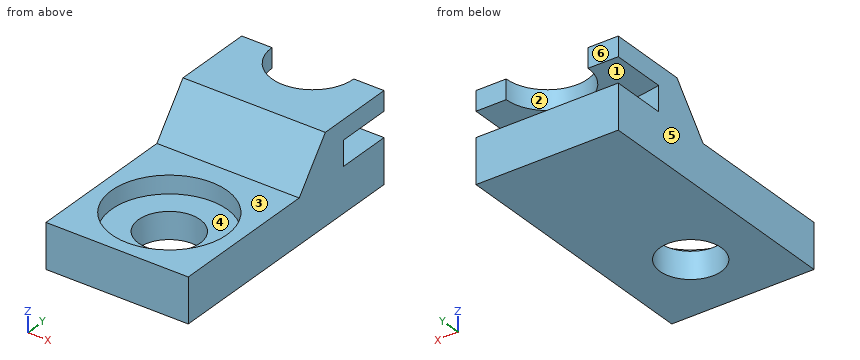
```python
from build123d import *

# Parameters (mm, degrees)
F0_W           = 10.16
F0_H           = 19.05
F1_DEPTH       = 3.175
F4_DEPTH       = 10.16
F6_D           = 4.4
F6_DEPTH       = 12.7
F6_CBORE_D     = 8.25
F6_CBORE_DEPTH = 1.27
F7_R           = 25.4
F8_DEPTH       = 1.778
F9_R           = 2.921
F10_DEPTH      = 2.54


with BuildPart() as f1:
    # F0 (on Top) → F1 (new body)
    with BuildSketch(Plane.XY):
        Rectangle(F0_W, F0_H)
    extrude(amount=F1_DEPTH)

    # F2 (on face) → F4 (join, through all)
    with BuildSketch(Plane.YZ.offset(5.08)):
        Polygon((3.81, 6.35), (1.27, 3.175), (9.525, 3.175), (9.525, 6.35), align=None)
    extrude(amount=-F4_DEPTH)

    # F6
    with Locations(Plane.XY.offset(3.175)):
        with Locations((0, -4.445)):
            CounterBoreHole(F6_D / 2, F6_CBORE_D / 2, F6_CBORE_DEPTH, depth=F6_DEPTH)

    # F7 (on face) → F8 (cut)
    with BuildSketch(Plane.XY.offset(3.175)):
        with Locations((0, 30.48)):
            Circle(F7_R)
    extrude(amount=F8_DEPTH, mode=Mode.SUBTRACT)

    # F9 (on face) → F10 (cut)
    with BuildSketch(Plane.XY.offset(6.35)):
        with Locations((0, 9.525)):
            Circle(F9_R)
    extrude(amount=-F10_DEPTH, mode=Mode.SUBTRACT)


solid = f1.part
```
Input: part model. Units: mm. Frame: model coordinates. Face numbers are marked on the shaded views. A direction names the side the tool comes from. Round coordinates to 2 decimals unless told otherwise and drop trailing zeros. Loops run counter-clockwise (first coordinate to the right, second up) from the corner with the lowest first, then second, coordinate; pieces in that order, holes last. Notation, with made-up numbers: (72.5, 60) -> (98.5, 60) arc R8 ccw to (98.5, 73) -> close; hole circle Ø8 at (84, -26.5). An arc over 180 degrees is marked (long way). Write each question's results on one line, items separated by ' | '.
1. Mould query, pull axis Y, two halves, no side actions, for the marked faces 4, 5 and 6. Classes: +Y half, -Y half, draft (parallel to the pull), parting line (faces both ways), or undercut.
Geometry results:
face 4: undercut | face 5: draft | face 6: +Y half
2. First-contact query: P1, Ø4, axis at x = 0, y = -4.5, coming from the +Z side; P2, Ø5, axis at x = 1.5, y = -6.5, coming from the +Z side (3 decimals). Flat tips, straight axial feed; report the tip coordinate or a pass-through.
Geometry results:
P1: through | P2: z = 3.175
3. Section C-C (x = -3.5). Return loops of the section in (y, z) (3 decimals), and give its area (3 significant figures).
Geometry results:
outline: (-9.525, 0) -> (9.525, 0) -> (9.525, 3.175) -> (5.322, 3.175) -> (5.322, 4.953) -> (9.525, 4.953) -> (9.525, 6.35) -> (3.81, 6.35) -> (1.27, 3.175) -> (-2.262, 3.175) -> (-2.262, 1.905) -> (-6.628, 1.905) -> (-6.628, 3.175) -> (-9.525, 3.175) -> close | area: 69.6 mm2
4. Section B-B (y = 7.5). Return loops of the section in (x, z) (3 decimals).
Geometry results:
outline: (-5.08, 0) -> (5.08, 0) -> (5.08, 3.175) -> (-5.08, 3.175) -> close; (-5.08, 4.953) -> (-2.105, 4.953) -> (-2.105, 6.35) -> (-5.08, 6.35) -> close; (2.105, 4.953) -> (5.08, 4.953) -> (5.08, 6.35) -> (2.105, 6.35) -> close
5. Ray query, line 1 (Z direction, x = 4.5, y = -4.75) (3 decimals); line 2 (Y direction, x = 0, z = 0.5) (3 decimals); line 3 (Y direction, x = -3.25, z = 2.75) (3 decimals). Return the intervals inside material, ascending. Write a range as from..to.
Geometry results:
line 1: 0..3.175 | line 2: -9.525..-6.645, -2.245..9.525 | line 3: -9.525..-6.985, -1.905..9.525
6. Set-up query: the marked faces 1, 2 and 3. Return all of +Z, -Z, +X, -X, +Y, -Y with unobstructed straight access to the full face (end or side cutting, diameter ignored); none if empty.
Geometry results:
face 1: +Y | face 2: +Z, +Y | face 3: +Z, +X, -X, -Y
7. Section D-D (y = -1.5). Return loops of the section in (x, z) (3 decimals).
Geometry results:
outline: (-5.08, 0) -> (5.08, 0) -> (5.08, 3.175) -> (2.888, 3.175) -> (2.888, 1.905) -> (-2.888, 1.905) -> (-2.888, 3.175) -> (-5.08, 3.175) -> close
8. Section A-A (x = 0). Return loops of the section in (y, z) (3 decimals).
Geometry results:
outline: (-9.525, 0) -> (-6.645, 0) -> (-6.645, 1.905) -> (-8.57, 1.905) -> (-8.57, 3.175) -> (-9.525, 3.175) -> close; (-2.245, 0) -> (9.525, 0) -> (9.525, 3.175) -> (5.08, 3.175) -> (5.08, 4.953) -> (6.604, 4.953) -> (6.604, 6.35) -> (3.81, 6.35) -> (1.27, 3.175) -> (-0.32, 3.175) -> (-0.32, 1.905) -> (-2.245, 1.905) -> close
